```python
from build123d import *

# Parameters (mm, degrees)
SKETCH1_W           = 71.12
SKETCH1_H           = 142.24
SKETCH1_W_2         = 17.145
SKETCH1_H_2         = 6.35
SKETCH1_W_3         = 6.35
SKETCH1_H_3         = 25.4
BOSS_EXTRUDE1_DEPTH = 6.35


with BuildPart() as part:
    # Sketch1 → Boss-Extrude1 (new body)
    with BuildSketch(Plane.XY):
        Rectangle(SKETCH1_W, SKETCH1_H)
        Polygon((35.56, -81.28), (35.56, -71.12), (0, -71.12), (0, -116.84), (9.2075, -116.84), (26.3525, -116.84), (35.56, -116.84), (35.56, -106.68), align=None)
        with Locations((17.78, -120.015)):
            Rectangle(SKETCH1_W_2, SKETCH1_H_2)
        with Locations((38.735, 58.42)):
            Rectangle(SKETCH1_W_3, SKETCH1_H_3)
        with Locations((38.735, 7.62)):
            Rectangle(SKETCH1_W_3, SKETCH1_H_3)
        with Locations((38.735, -43.18)):
            Rectangle(SKETCH1_W_3, SKETCH1_H_3)
        with Locations((38.735, -93.98)):
            Rectangle(SKETCH1_W_3, SKETCH1_H_3)
        with Locations((-38.735, -43.18)):
            Rectangle(SKETCH1_W_3, SKETCH1_H_3)
        with Locations((-38.735, 7.62)):
            Rectangle(SKETCH1_W_3, SKETCH1_H_3)
        with Locations((-38.735, 58.42)):
            Rectangle(SKETCH1_W_3, SKETCH1_H_3)
    extrude(amount=BOSS_EXTRUDE1_DEPTH)


solid = part.part
```
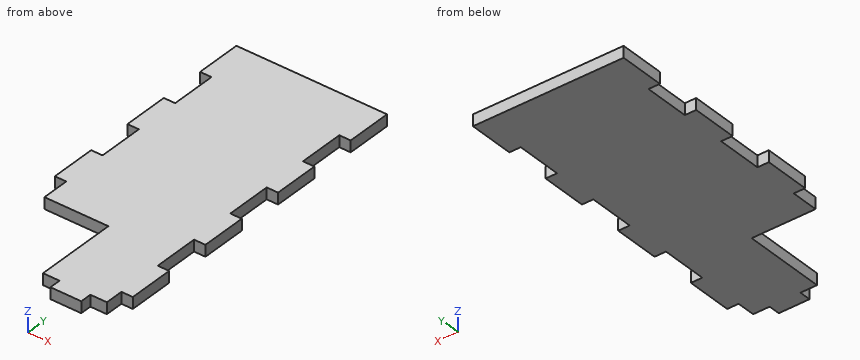
Input: part model. Units: mm. Frame: model coordinates. Coordinates: 2 decimals unless noted, no trailing zeros. Loops run counter-clockwise (first coordinate to the right, second up) from the corner with the lowest first, then second, coordinate; pieces in that order, holes last.
Q1. Contact query for flat-ended pins moving along their axis: pin 1 (3 mm diameter, centred on x = -15.5, y = 32.5, fed in from -Z); pin 2 (3 mm diameter, centred on y = -87, z = 2.5, fed in from -X); pin 3 (3 mm diameter, centred on x = 28.5, z = 2, fed in from -Y). Output: stop coordinate, or through.
Results are:
pin 1: stops at z = 0
pin 2: stops at x = 0
pin 3: stops at y = -116.84
Q2. Section B-B, the plane x = -20. Return the cut outline in (y, z), and give its area (3 significant figures).
Results are:
outline: (-71.12, 0) - (71.12, 0) - (71.12, 6.35) - (-71.12, 6.35) - close
area: 903 mm2
Q3. Line query: line 1 along Y through (x, z) = (33, 6); line 2 along Y through (x, z) = (-28, 1.25); line 3 along X through (y, z) = (-76, 6). Output: solid intervals per line, ascending.
Results are:
line 1: y = -116.84 to 71.12
line 2: y = -71.12 to 71.12
line 3: x = 0 to 35.56
Q4. Section C-C, the plane y = -99. Return the cut outline in (x, z).
Results are:
outline: (0, 0) - (41.91, 0) - (41.91, 6.35) - (0, 6.35) - close
